from build123d import *

# Parameters (mm, degrees)
SKETCH052_R     = 2.7
PAD038_DEPTH    = 19
PAD039_DEPTH    = 17.74
SKETCH053_R     = 0.95
POCKET009_DEPTH = 8.3
SKETCH081_R     = 0.95
POCKET025_DEPTH = 8


with BuildPart() as part:
    # Sketch052 (on ShapeBinder) → Pad038 (new body)
    with BuildSketch(Plane(origin=(0, 0, 0), x_dir=(-1, 0, 0), z_dir=(0, 0, 1))):
        with Locations((0, 37.1)):
            Circle(SKETCH052_R)
    extrude(amount=PAD038_DEPTH)

    # Sketch052 (on ShapeBinder) → Pad039 (join)
    with BuildSketch(Plane(origin=(0, 0, 0), x_dir=(-1, 0, 0), z_dir=(0, 0, 1))):
        with Locations((0, 37.1)):
            Circle(SKETCH052_R)
    extrude(amount=-PAD039_DEPTH)

    # Sketch053 (on Face1 of Pad039) → Pocket009 (cut)
    with BuildSketch(Plane(origin=(0, 0, -17.74), x_dir=(1, 0, 0), z_dir=(0, 0, -1))):
        with Locations((0, 37.1)):
            Circle(SKETCH053_R)
        with BuildLine():
            Line((-1.8, 35.0875388203), (-1.8, 39.1124611797))
            ThreePointArc((-1.8, 39.1124611797), (-2.7, 37.1), (-1.8, 35.0875388203))
        make_face()
        with BuildLine():
            Line((1.8, 39.1124611797), (1.8, 35.0875388203))
            ThreePointArc((1.8, 35.0875388203), (2.7, 37.1), (1.8, 39.1124611797))
        make_face()
    extrude(amount=-POCKET009_DEPTH, mode=Mode.SUBTRACT)

    # Sketch081 (on Face8 of Pocket009) → Pocket025 (cut)
    with BuildSketch(Plane(origin=(0, 0, 19), x_dir=(-1, 0, 0), z_dir=(0, 0, 1))):
        with Locations((0, 37.1)):
            Circle(SKETCH081_R)
        with BuildLine():
            ThreePointArc((-1.8, 39.1124611797), (-2.7, 37.1), (-1.8, 35.0875388203))
            Line((-1.8, 39.1124611797), (-1.8, 35.0875388203))
        make_face()
        with BuildLine():
            Line((1.8, 39.1124611797), (1.8, 35.0875388203))
            ThreePointArc((1.8, 35.0875388203), (2.7, 37.1), (1.8, 39.1124611797))
        make_face()
    extrude(amount=-POCKET025_DEPTH, mode=Mode.SUBTRACT)


with BuildPart() as part_1:
    # Body024 placement: moved
    add(part.part.moved(Location((0, 37.1, 0))))


solid = part_1.part
CAD build for the part. Positions are in the model's coordinates, mm. A direction names the side the tool comes from. Coordinates: 2 decimals unless noted, no trailing zeros. Loops run counter-clockwise (first coordinate to the right, second up) from the corner with the lowest first, then second, coordinate; pieces in that order, holes last. Notation, with made-up numbers: (57, 87) -> (64, 87) arc R28 cw to (64, 106) -> close; hole circle Ø10 at (18.25, -18). An arc over 180 degrees is marked (long way). One line per item, written item: value.
1. Slice it at B-B on y = 0. Write the cut outline in (x, z).
Answers:
outline: (-2.7, -9.44) -> (-1.8, -9.44) -> (-1.8, -17.74) -> (-0.95, -17.74) -> (-0.95, -9.44) -> (0.95, -9.44) -> (0.95, -17.74) -> (1.8, -17.74) -> (1.8, -9.44) -> (2.7, -9.44) -> (2.7, 11) -> (1.8, 11) -> (1.8, 19) -> (0.95, 19) -> (0.95, 11) -> (-0.95, 11) -> (-0.95, 19) -> (-1.8, 19) -> (-1.8, 11) -> (-2.7, 11) -> close
2. Slice it at A-A on x = 0. Write the cut outline in (y, z).
Answers:
outline: (-2.7, -17.74) -> (-0.95, -17.74) -> (-0.95, -9.44) -> (0.95, -9.44) -> (0.95, -17.74) -> (2.7, -17.74) -> (2.7, 19) -> (0.95, 19) -> (0.95, 11) -> (-0.95, 11) -> (-0.95, 19) -> (-2.7, 19) -> close
3. Slice it at D-D on y = 1.55. Write the cut outline in (x, z), and give its area (3 significant figures).
Answers:
outline: (-2.21, -9.44) -> (-1.8, -9.44) -> (-1.8, -17.74) -> (1.8, -17.74) -> (1.8, -9.44) -> (2.21, -9.44) -> (2.21, 11) -> (1.8, 11) -> (1.8, 19) -> (-1.8, 19) -> (-1.8, 11) -> (-2.21, 11) -> close
area: 149 mm^2
4. Pull direction X, two halves, no side cores. Call faces 5 (the face through (1.8, 0, 15)), 6 (the face through (2, 0, 11)), 7 (the face through (0, 0, 11)): pulls with the +X half, pulls with the -X half, needs draft (parallel to the pull), parting line crosses it, or undercut.
Answers:
face 5: pulls with the +X half
face 6: needs draft
face 7: undercut
5. Which spindle directions (+Z, -Z, +X, -X, +Y, -Y) get a long thin tool onto all of the face, cutting with end or side? Do faces 1 (the face through (1.8, 0, -14)), 2 (the face through (0, 0, -9.44)), 3 (the face through (-2, 0, -9.44)), 4 (the face through (-1.8, 0, 15)). Say none if no direction does.
Answers:
face 1: -Z, +X, +Y, -Y
face 2: -Z
face 3: -Z, -X, +Y, -Y
face 4: +Z, -X, +Y, -Y
6. Slice it at C-C on z = 0. Write the cut outline in (x, y).
Answers:
outline: circle Ø5.4 at (0, 0)
7. Drill centre lines: line 1 (X direction, y = 0, z = 15); line 2 (Y direction, x = 0, z = -16); line 3 (Z direction, x = -2.1, y = -0.9). Where is each one in solid material? Low to high. Write a range as [from, to].
Answers:
line 1: x = [-1.8, -0.95], [0.95, 1.8]
line 2: y = [-2.7, -0.95], [0.95, 2.7]
line 3: z = [-9.44, 11]
8. Flat gauge pins, fed straight in: P1, Ø1.1, axis at x = 0, y = 0, coming from the +Z side; P2, Ø1.2, axis at y = -0.5, z = 14.5, coming from the +X side; P3, Ø3, axis at y = 1, z = 14, coming from the -X side. Where does each tip first touch, or does it go through?
Answers:
P1: stops at z = 11
P2: stops at x = 1.8
P3: stops at x = -1.8
